Read the model definition and answer for the solid it produces. Units are mm, in the model's axes. A direction names the side the tool comes from. Round coordinates to 2 decimals unless told otherwise and drop trailing zeros. Loops run counter-clockwise (first coordinate to the right, second up) from the corner with the lowest first, then second, coordinate; pieces in that order, holes last. Notation, with made-up numbers: (51, 10) - (58, 10) arc R17 cw to (58, 36) - close; hole circle Ø5 at (19.25, 20.25). An arc over 180 degrees is marked (long way). Use CSV: the item, a comma, the result in double quotes. Start each with the question number.
1. Given pin 1 Ø0.9 at (y, z) = (31, 2) entering from -X; pin 2 Ø1.5 at (x, z) = (-14, 1.5) entering from +Y; pin 3 Ø3 at (x, y) = (42.1, 56.79) entering from -Z; pin 4 Ø0.9 at (y, z) = (14, 1.5) entering from +X, each flat-ended and moving along its own axis, determine where each tip first touches the part or whether it passes through.
2. Consider line 1 along X through (y, z) = (10.5, 1.35); line 2 along Y through (x, z) = (-27, 1.9); line 3 along X through (y, z) = (24.5, 0.8). Determine where each line is inside the solid, lowest interval first.
3. Find section D-D (z = 0.9). State how many separate pieces and enclosed holes the cut face has, and give its area (3 significant figures).
4. Determine the mould class of faces 1 (the flat face through (49.706, -14.607, 1.479)), 2 (the cylindrical face through (20.4, 50.69, 1.48)), 3 (the flat face through (37, 71.788, 1)) for opening direction Y: +Y half, -Y half, draft (parallel to the pull), parting line (faces both ways), or undercut.
5. A tool of negligible diameter and unlimited length cuts with its end or side. For faces 4 (the flat face through (49.999, 25, 1)), 5 (the cylindrical face through (43.685, 0.53, 1.479)), 6 (the flat face through (-36.46, 67.35, 1.48)), 7 (the flat face through (-4, 15, 3)), 8 (the flat face through (-59.371, 24, 1)), from which of +Z, -Z, +X, -X, +Y, -Y can it reach the whole face along a straight path? Write none if from no direction.
6. Find section C-C (y = 31). Give the vertices of the cut face in (x, z).
7. Find section B-B (x = -5.5). Give the vertices of the cut face in (y, z), and give its area (3 significant figures).
8. Find section A-A (x = 11.5). Give the vertices of the cut face in (y, z).
from build123d import *

# Parameters (mm, degrees)
SKETCH1_R           = 7.50000053
SKETCH1_R_2         = 1.6
BOSS_EXTRUDE1_DEPTH = 3


with BuildPart() as part:
    # Sketch1 → Boss-Extrude1 (new body)
    with BuildSketch(Plane.XY):
        Polygon((-66.89924788, 56.788402458), (-51.89924788, 71.788403422), (-40.89924788, 71.788403422), (-31.89924788, 62.788403422), (22.10075212, 62.788403422), (31.10075212, 71.788403422), (42.10075212, 71.788403422), (57.10075212, 56.788402458), (49.999134038, 47.546675265), (49.999134038, 2.030197685), (57.10075212, -7.211596578), (42.10075212, -22.211596578), (31.10075212, -22.211596578), (22.10075212, -20.180597469), (-31.89924788, -20.180597469), (-40.89924788, -22.211598699), (-51.89924788, -22.211598699), (-66.89924788, -7.211596578), (-59.371431864, 2.030197685), (-59.371431864, 47.546675265), align=None)
        with Locations((-4.89924788, 24.798725856)):
            Circle(SKETCH1_R, mode=Mode.SUBTRACT)
        with Locations((-51.89924788, 56.788403422)):
            Circle(SKETCH1_R_2, mode=Mode.SUBTRACT)
        with Locations((42.10075212, 56.788403422)):
            Circle(SKETCH1_R_2, mode=Mode.SUBTRACT)
        with Locations((42.10075212, -7.211596578)):
            Circle(SKETCH1_R_2, mode=Mode.SUBTRACT)
        with Locations((-51.89924788, -7.211596578)):
            Circle(SKETCH1_R_2, mode=Mode.SUBTRACT)
        with BuildLine():
            Line((-47.943404379, 50.293594248), (-46.443406464, 50.296157806))
            ThreePointArc((-46.443406464, 50.296157806), (-44.318775436, 49.419295137), (-43.438283518, 47.296165805))
            Line((-43.438283518, 47.296165805), (-43.438283518, 2.301285908))
            ThreePointArc((-43.438283518, 2.301285908), (-44.312414708, 0.171678429), (-46.438272777, -0.711532092))
            Line((-46.438272777, -0.711532092), (-47.938272883, -0.711532092))
            ThreePointArc((-47.938272883, -0.711532092), (-50.059593376, 0.167147627), (-50.938273095, 2.28846812))
            Line((-50.938273095, 2.28846812), (-50.938273095, 47.288471302))
            ThreePointArc((-50.938273095, 47.288471302), (-50.063220077, 49.411290395), (-47.943404379, 50.293594248))
        make_face(mode=Mode.SUBTRACT)
        with BuildLine():
            Line((-28.054738716, 57.288403953), (18.256242957, 57.288403953))
            ThreePointArc((18.256242957, 57.288403953), (20.377563451, 56.409724234), (21.256243169, 54.28840374))
            Line((21.256243169, 54.28840374), (21.256243169, 52.788403634))
            ThreePointArc((21.256243169, 52.788403634), (20.377563451, 50.667083141), (18.256242957, 49.788403422))
            Line((18.256242957, 49.788403422), (-28.054738716, 49.788403422))
            ThreePointArc((-28.054738716, 49.788403422), (-30.17605921, 50.667083141), (-31.054738929, 52.788403634))
            Line((-31.054738929, 52.788403634), (-31.054738929, 54.28840374))
            ThreePointArc((-31.054738929, 54.28840374), (-30.17605921, 56.409724234), (-28.054738716, 57.288403953))
        make_face(mode=Mode.SUBTRACT)
        with BuildLine():
            Line((40.986432116, 50.152198784), (39.487237783, 50.201358441))
            ThreePointArc((39.487237783, 50.201358441), (37.338259765, 49.392672987), (36.390529804, 47.30128909))
            Line((36.390529804, 47.30128909), (36.390529804, 2.296162622))
            ThreePointArc((36.390529804, 2.296162622), (37.63815416, -0.88414715), (41.054067708, -0.834433807))
            Line((41.054067708, -0.834433807), (42.553262041, -0.78527415))
            ThreePointArc((42.553262041, -0.78527415), (43.695191197, 0.55294834), (43.890530335, 2.301285908))
            Line((43.890530335, 2.301285908), (43.890530335, 47.30128909))
            ThreePointArc((43.890530335, 47.30128909), (42.995792019, 49.294452303), (40.986432116, 50.152198784))
        make_face(mode=Mode.SUBTRACT)
        with BuildLine():
            Line((18.778253795, -14.680597999), (-28.576749554, -14.680597999))
            ThreePointArc((-28.576749554, -14.680597999), (-30.698070048, -13.801918281), (-31.576749766, -11.680597787))
            Line((-31.576749766, -11.680597787), (-31.576749766, -10.180597681))
            ThreePointArc((-31.576749766, -10.180597681), (-30.698070048, -8.059277188), (-28.576749554, -7.180597469))
            Line((-28.576749554, -7.180597469), (18.778253795, -7.180597469))
            ThreePointArc((18.778253795, -7.180597469), (20.899574288, -8.059277188), (21.778254007, -10.180597681))
            Line((21.778254007, -10.180597681), (21.778254007, -11.680597787))
            ThreePointArc((21.778254007, -11.680597787), (20.899574288, -13.801918281), (18.778253795, -14.680597999))
        make_face(mode=Mode.SUBTRACT)
    extrude(amount=BOSS_EXTRUDE1_DEPTH)


solid = part.part
Filled sheet:
1,pin 1,"stops at x = -59.37"
1,pin 2,"stops at y = 62.79"
1,pin 3,"passes through"
1,pin 4,"stops at x = 50"
2,line 1,"x = -59.37 to -50.94, -43.44 to 36.39, 43.89 to 50"
2,line 2,"y = -20.18 to -14.68, -7.18 to 49.79, 57.29 to 62.79"
2,line 3,"x = -59.37 to -50.94, -43.44 to -12.39, 2.59 to 36.39, 43.89 to 50"
3,separate pieces,"1"
3,enclosed holes,"9"
3,area,"7,970 mm²"
4,face 1,"-Y half"
4,face 2,"undercut"
4,face 3,"+Y half"
5,face 4,"+Z, -Z, +X"
5,face 5,"+Z, -Z"
5,face 6,"+Z, -Z, +Y"
5,face 7,"+Z, +X, -X, +Y, -Y"
5,face 8,"+Z, -Z, -X"
6,outline,"(-59.37, 0) - (-50.94, 0) - (-50.94, 3) - (-59.37, 3) - close; (-43.44, 0) - (-9.12, 0) - (-9.12, 3) - (-43.44, 3) - close; (-0.68, 0) - (36.39, 0) - (36.39, 3) - (-0.68, 3) - close; (43.89, 0) - (50, 0) - (50, 3) - (43.89, 3) - close"
7,outline,"(-20.18, 0) - (-14.68, 0) - (-14.68, 3) - (-20.18, 3) - close; (-7.18, 0) - (17.32, 0) - (17.32, 3) - (-7.18, 3) - close; (32.27, 0) - (49.79, 0) - (49.79, 3) - (32.27, 3) - close; (57.29, 0) - (62.79, 0) - (62.79, 3) - (57.29, 3) - close"
7,area,"159 mm²"
8,outline,"(-20.18, 0) - (-14.68, 0) - (-14.68, 3) - (-20.18, 3) - close; (-7.18, 0) - (49.79, 0) - (49.79, 3) - (-7.18, 3) - close; (57.29, 0) - (62.79, 0) - (62.79, 3) - (57.29, 3) - close"
